Could you check a few things on this model? Use its own coordinates, in mm. A direction names the side the tool comes from. Round coordinates to 2 decimals unless told otherwise and drop trailing zeros. Loops run counter-clockwise (first coordinate to the right, second up) from the corner with the lowest first, then second, coordinate; pieces in that order, holes last. Notation, with made-up numbers: (89, 14.5) -> (111, 14.5) arc R33 ccw to (111, 53.5) -> close; hole circle Ø7 at (-34.75, 73). An arc over 180 degrees is marked (long way). One line per item, written item: value.
Autodesk Inventor part; units mm, degrees
ref_plane "YZ Plane" through (0, 0, 0) normal (1, 0, 0) x (0, 1, 0)
ref_plane "XZ Plane" through (0, 0, 0) normal (0, 1, 0) x (-1, 0, 0)
ref_plane "XY Plane" through (0, 0, 0) normal (0, 0, 1) x (1, 0, 0)
sketch "Sketch1" plane through (0, 0, 0) normal (0, 1, 0) x (-1, 0, 0)
  arc A0 (0, -69.85) -> (65.9911, -22.8953) centre (0, 0) ccw
  line L0 (0, 0) -> (60.4919, -34.925)
  line L1 (0, 0) -> (69.85, 0) construction
  line L2 (60.4919, -34.925) -> (82.4889, -47.625)
  line L3 (60.4919, -34.925) -> (71.4904, -41.275)
  line L4 (60.4919, -34.925) -> (60.4919, -47.625)
  line L5 (60.4919, -47.625) -> (82.4889, -47.625)
  line L6 (60.4919, -34.925) -> (82.4889, -34.925)
  line L7 (82.4889, -34.925) -> (82.4889, -47.625)
  line L8 (82.4889, -34.925) -> (60.4919, -47.625)
  circle A1 centre (71.4904, -41.275) radius 9.779
  circle A2 centre (71.4904, -41.275) radius 3.175
  circle A3 centre (71.4904, -51.054) radius 2.286
  circle A4 centre (71.4904, -31.496) radius 2.286
  circle A5 centre (81.2694, -41.275) radius 2.286
  circle A6 centre (61.7114, -41.275) radius 2.286
  line L9 (65.9911, -22.8953) -> (91.3911, -22.8953)
  line L10 (91.3911, -22.8953) -> (91.3911, -60.9953)
  line L11 (91.3911, -60.9953) -> (33.2947, -60.9953)
  line L12 (0, 0) -> (0, -69.85)
  line L13 (0, 0) -> (65.9911, -22.8953)
  line L14 (0, -69.85) -> (0, -76.585)
  line L15 (0, -76.585) -> (45.4402, -60.9953)
  dimension "d0" = 139.7
  dimension "d1" = 30
  dimension "d2" = 25.4
  dimension "d3" = 19.558
  dimension "d4" = 6.35
  dimension "d5" = 4.572
  dimension "d6" = 4.572
  dimension "d7" = 4.572
  dimension "d8" = 4.572
  dimension "d9" = 25.4
  dimension "d10" = 38.1
extrude "Extrusion1" add sketch "Sketch1" along normal blind 12.7 contours A0 L9 L10 L11 | L6 A1 L2 | L2 A1 A6 L4 | L11 L15 L14 A0 | A1 L6 L8 A2 L2 | L2 A2 L8 A1 A6 | A1 A4 L6 | A6 A1 L8 L4 | L6 L8 A1 | L8 A1 A5 L2 A2 | A2 L2 A1 L5 L8 | L8 A1 L5 | L7 A5 A1 L8 | L5 A1 A3 | A1 A5 L7 L2 | L2 L5 A1
properties part number "NewShooterFlicker"
(1) If we section it at B-B, the plane x = -8: Please give me the cut outline in (y, z).
Recorded:
outline: (0, -73.84) -> (12.7, -73.84) -> (12.7, -69.39) -> (0, -69.39) -> close
(2) If we section it at A-A, the plane y = 11.25: Please give me the cut outline in (x, z) (3 decimals), then the cut area to 3 significant figures.
Recorded:
outline: (-91.391, -60.995) -> (-45.44, -60.995) -> (0, -76.585) -> (0, -69.85) arc R69.85 cw to (-65.991, -22.895) -> (-91.391, -22.895) -> close; hole circle Ø4.572 at (-81.269, -41.275); hole circle Ø6.35 at (-71.49, -41.275); hole circle Ø4.572 at (-71.49, -51.054); hole circle Ø4.572 at (-71.49, -31.496); hole circle Ø4.572 at (-61.711, -41.275)
area: 1,480 mm²
(3) Thinking about a two-plate mould opening in Z: for faces 1 (the face through (-66, 12.7, -48)), 2 (the face through (-22.4, 6.3, -68.9)), 3 (the face through (-40.99, 6.26, -56.56)), 4 (the face through (-61.216, 6.261, -39.043)), which applies, released by +Z, released by -Z, zero draft, split by the parting line, or undercut?
Recorded:
face 1: zero draft
face 2: released by -Z
face 3: released by +Z
face 4: undercut
(4) If I drill on L1, parallel to Z at x = -81.5, y = 5.25; L2, parallel to X at y = 8.25, z = -30; L3, parallel to Z at x = -62.5, y = 10.5, over which ranges is the centre line in solid material (lowest first)?
Recorded:
L1: -61 to -43.55, -39 to -22.9
L2: -91.39 to -73.22, -69.76 to -63.08
L3: -61 to -43.42, -39.13 to -31.19
(5) For faces 5 (the face through (-79.46, 6.26, -39.88)), 6 (the face through (-69, 6, -60.995)), which set-ups out of +Z, -Z, +X, -X, +Y, -Y let a thin tool reach every point of the face, with its end or its side?
Recorded:
face 5: +Y, -Y
face 6: -Z, -X, +Y, -Y
(6) If we section it at C-C, the plane z = -73: Please give me the cut outline in (x, y), then the cut area to 3 significant figures.
Recorded:
outline: (-10.45, 0) -> (0, 0) -> (0, 12.7) -> (-10.45, 12.7) -> close
area: 133 mm²
(7) I'm going to push flat-ended pins straight in: pin 1 Ø5 at (x, y) = (-59.5, 3) entering from -Z; pin 2 Ø2 at (x, y) = (-55, 9.5) entering from +Z; pin 3 Ø4 at (x, y) = (-20.5, 10.5) entering from +Z. Where does each tip first touch, or does it pass through?
Recorded:
pin 1: z = -61
pin 2: z = -41.75
pin 3: z = -66.13
